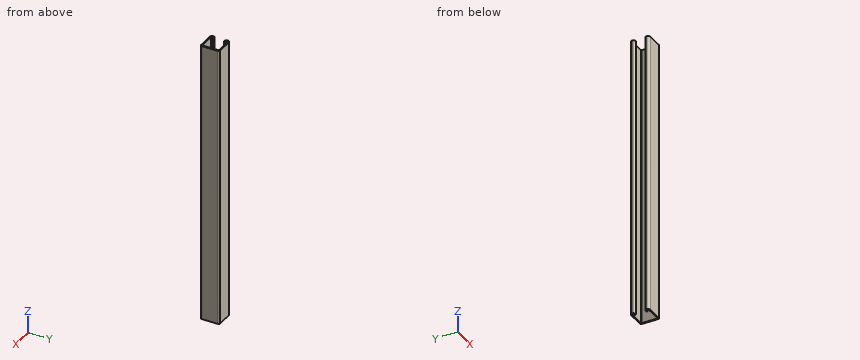
from build123d import *

# Parameters (mm, degrees)
BOSS_EXTRUDE1_DEPTH = 609.6


with BuildPart() as part:
    # Sketch1 → Boss-Extrude1 (new body)
    with BuildSketch(Plane.XY):
        with BuildLine():
            Line((-36.22675, 20.6375), (-3.46075, 20.6375))
            ThreePointArc((-3.46075, 20.6375), (-1.013630207, 19.623869793), (0, 17.17675))
            Line((0, 17.17675), (0, -17.17675))
            ThreePointArc((0, -17.17675), (-1.013630207, -19.623869793), (-3.46075, -20.6375))
            Line((-3.46075, -20.6375), (-36.22675, -20.6375))
            ThreePointArc((-36.22675, -20.6375), (-39.796401808, -19.158901808), (-41.275, -15.58925))
            Line((-41.275, -15.58925), (-41.275, -14.57325))
            ThreePointArc((-41.275, -14.57325), (-40.261369793, -12.126130207), (-37.81425, -11.1125))
            Line((-37.81425, -11.1125), (-35.5346, -11.1125))
            ThreePointArc((-35.5346, -11.1125), (-34.1376, -12.5095), (-35.5346, -13.9065))
            Line((-35.5346, -13.9065), (-37.81425, -13.9065))
            ThreePointArc((-37.81425, -13.9065), (-38.285713446, -14.101786554), (-38.481, -14.57325))
            Line((-38.481, -14.57325), (-38.481, -15.58925))
            ThreePointArc((-38.481, -15.58925), (-37.820745461, -17.183245461), (-36.22675, -17.8435))
            Line((-36.22675, -17.8435), (-3.46075, -17.8435))
            ThreePointArc((-3.46075, -17.8435), (-2.989286554, -17.648213446), (-2.794, -17.17675))
            Line((-2.794, -17.17675), (-2.794, 17.17675))
            ThreePointArc((-2.794, 17.17675), (-2.989286554, 17.648213446), (-3.46075, 17.8435))
            Line((-3.46075, 17.8435), (-36.22675, 17.8435))
            ThreePointArc((-36.22675, 17.8435), (-37.820745461, 17.183245461), (-38.481, 15.58925))
            Line((-38.481, 15.58925), (-38.481, 14.57325))
            ThreePointArc((-38.481, 14.57325), (-38.285713446, 14.101786554), (-37.81425, 13.9065))
            Line((-37.81425, 13.9065), (-35.5346, 13.9065))
            ThreePointArc((-35.5346, 13.9065), (-34.1376, 12.5095), (-35.5346, 11.1125))
            Line((-35.5346, 11.1125), (-37.81425, 11.1125))
            ThreePointArc((-37.81425, 11.1125), (-40.261369793, 12.126130207), (-41.275, 14.57325))
            Line((-41.275, 14.57325), (-41.275, 15.58925))
            ThreePointArc((-41.275, 15.58925), (-39.796401808, 19.158901808), (-36.22675, 20.6375))
        make_face()
    extrude(amount=-BOSS_EXTRUDE1_DEPTH)


solid = part.part
CAD build for the part. Positions are in the model's coordinates, mm. Round coordinates to 2 decimals unless told otherwise and drop trailing zeros. Write each loop counter-clockwise with the first axis right and the second up, starting at its lowest first coordinate (ties: lowest second). Pieces come first, ordered by that corner, then holes. Notation, with made-up numbers: (-29.5, -3) -> (18.5, -3) arc R18 ccw to (18.5, 4) -> close; hole circle Ø11 at (24, 81). An arc over 180 degrees is marked (long way). Answer as a JSON object with one key per item and string values.
(1) Band-saw the part on B-B, the plane z = -347.5. List the corners of the cut face in (x, y) (1 decimal), then the cut area to 3 significant figures.
Reported:
{"outline": "(-41.3, -15.6) arc R5 ccw to (-36.2, -20.6) -> (-3.5, -20.6) arc R3.5 ccw to (0, -17.2) -> (0, 17.2) arc R3.5 ccw to (-3.5, 20.6) -> (-36.2, 20.6) arc R5 ccw to (-41.3, 15.6) -> (-41.3, 14.6) arc R3.5 ccw to (-37.8, 11.1) -> (-35.5, 11.1) arc R1.4 ccw to (-35.5, 13.9) -> (-37.8, 13.9) arc R0.7 cw to (-38.5, 14.6) -> (-38.5, 15.6) arc R2.3 cw to (-36.2, 17.8) -> (-3.5, 17.8) arc R0.7 cw to (-2.8, 17.2) -> (-2.8, -17.2) arc R0.7 cw to (-3.5, -17.8) -> (-36.2, -17.8) arc R2.3 cw to (-38.5, -15.6) -> (-38.5, -14.6) arc R0.7 cw to (-37.8, -13.9) -> (-35.5, -13.9) arc R1.4 ccw to (-35.5, -11.1) -> (-37.8, -11.1) arc R3.5 ccw to (-41.3, -14.6) -> close", "area": "372 mm^2"}
(2) Pin check, flat tip, straight feed: P1, Ø12, axis at y = 3, z = -323, coming from the -X side. Stop position of the tip, or through.
Reported:
{"P1": "stops at x = -2.79"}
(3) Band-saw the part on C-C, the plane y = -5. List the corners of the cut face in (x, z).
Reported:
{"outline": "(-2.79, -609.6) -> (0, -609.6) -> (0, 0) -> (-2.79, 0) -> close"}
(4) Probe probe 1 along Y at (x, z) = (-35.5, -358); probe 2 along Y at (x, z) = (-12, -156); probe 3 along X at (y, z) = (1, -303). List the from-to ranges inside material, lowest first. Write a range as [from, to].
Reported:
{"probe 1": "y = [-20.64, -17.84], [-13.91, -11.11], [11.11, 13.91], [17.84, 20.64]", "probe 2": "y = [-20.64, -17.84], [17.84, 20.64]", "probe 3": "x = [-2.79, 0]"}
(5) Band-saw the part on A-A, the plane x = -12.5. List the corners of the cut face in (y, z), then the cut area to 3 significant figures.
Reported:
{"outline": "(-20.64, -609.6) -> (-17.84, -609.6) -> (-17.84, 0) -> (-20.64, 0) -> close; (17.84, -609.6) -> (20.64, -609.6) -> (20.64, 0) -> (17.84, 0) -> close", "area": "3,410 mm^2"}
